Autodesk Inventor part; units mm, degrees
ref_plane "YZ Plane" through (0, 0, 0) normal (1, 0, 0) x (0, 1, 0)
ref_plane "XZ Plane" through (0, 0, 0) normal (0, 1, 0) x (-1, 0, 0)
ref_plane "XY Plane" through (0, 0, 0) normal (0, 0, 1) x (1, 0, 0)
sketch "Sketch1" plane through (0, 0, 0) normal (0, 1, 0) x (-1, 0, 0)
  line L0 (49.53, 22.225) -> (-49.53, 22.225)
  line L1 (-49.53, 22.225) -> (-49.53, -22.225)
  line L2 (-49.53, -22.225) -> (49.53, -22.225)
  line L3 (49.53, -22.225) -> (49.53, 22.225)
  line L4 (49.53, 22.225) -> (-49.53, -22.225) construction
  line L5 (-49.53, 22.225) -> (49.53, -22.225) construction
  line L6 (50.53, 23.225) -> (-50.53, 23.225)
  line L7 (-50.53, 23.225) -> (-50.53, -23.225)
  line L8 (-50.53, -23.225) -> (50.53, -23.225)
  line L9 (50.53, -23.225) -> (50.53, 23.225)
  point P0 (0, 0)
  dimension "d0" = 44.45
  dimension "d1" = 99.06
  dimension "d2" = 1
extrude "Extrusion1" add sketch "Sketch1" along normal blind 6.35
chamfer "Chamfer1" distance 0.7937 angle 45 8 edges at (-50.53, 3.175, -23.225) (-49.53, 3.175, -22.225) (-49.53, 3.175, 22.225) (-50.53, 3.175, 23.225) (50.53, 3.175, -23.225) (49.53, 3.175, -22.225) (49.53, 3.175, 22.225) (50.53, 3.175, 23.225)
properties part number "band 18t" material "Rubber"
Check sheet for the modelled part. Datum: model origin and axes. Units: mm. A direction names the side the tool comes from. Coordinates: 2 decimals unless noted, no trailing zeros. Loops run counter-clockwise (first coordinate to the right, second up) from the corner with the lowest first, then second, coordinate; pieces in that order, holes last. Notation, with made-up numbers: (81, 78) -> (125, 78) arc R14 cw to (125, 85) -> close; hole circle Ø4 at (7, -6). An arc over 180 degrees is marked (long way). Write item = value, one per line. Start each with the question number.
1. Draft check along Z on faces 1 (the flat face through (-49.53, 3, 0)), 2 (the flat face through (1, 3, -23.225)), 3 (the flat face through (0.2, 6.35, 22.5)). Enter one of: released by +Z, released by -Z, zero draft, split by the parting line, or undercut.
2. Section check B-B on z = 16. Record the cut outline in (x, y), then the cut area to 3 significant figures.
3. Tool access check on faces 4 (the flat face through (-1, 3, 22.225)), 5 (the flat face through (-50.53, 3, 0)). Record the directions out of +Z, -Z, +X, -X, +Y, -Y that give a thin tool (end or side, any length) a straight path to the whole face; none if there is none.
4. Section check A-A on x = 38. Record the cut outline in (y, z) (3 decimals).
5. Material ranges on line 1 (X direction, y = 0.75, z = -17); line 2 (Z direction, x = 18, y = 4.75) (3 decimals), recorded low to high.
6. Section check C-C on y = 4.25. Record the cut outline in (x, z) (3 decimals).
Responses:
q1.face_1 = undercut
q1.face_2 = released by -Z
q1.face_3 = zero draft
q2.outline = (-50.53, 0) -> (-49.53, 0) -> (-49.53, 6.35) -> (-50.53, 6.35) -> close; (49.53, 0) -> (50.53, 0) -> (50.53, 6.35) -> (49.53, 6.35) -> close
q2.area = 12.7 mm2
q3.face_4 = +Y, -Y
q3.face_5 = +Z, -Z, -X, +Y, -Y
q4.outline = (0, -23.225) -> (6.35, -23.225) -> (6.35, -22.225) -> (0, -22.225) -> close; (0, 22.225) -> (6.35, 22.225) -> (6.35, 23.225) -> (0, 23.225) -> close
q5.line_1 = -50.53 to -49.53, 49.53 to 50.53
q5.line_2 = -23.225 to -22.225, 22.225 to 23.225
q6.outline = (-50.53, -22.431) -> (-49.736, -23.225) -> (49.736, -23.225) -> (50.53, -22.431) -> (50.53, 22.431) -> (49.736, 23.225) -> (-49.736, 23.225) -> (-50.53, 22.431) -> close; hole (-49.53, -21.431) -> (-48.736, -22.225) -> (48.736, -22.225) -> (49.53, -21.431) -> (49.53, 21.431) -> (48.736, 22.225) -> (-48.736, 22.225) -> (-49.53, 21.431) -> close
